Verification items for the finished model (mm, model axes). Face numbers are marked on the shaded views. A direction names the side the tool comes from. Round coordinates to 2 decimals unless told otherwise and drop trailing zeros. Loops run counter-clockwise (first coordinate to the right, second up) from the corner with the lowest first, then second, coordinate; pieces in that order, holes last.
from build123d import *

# Parameters (mm, degrees)
F3_DEPTH = 0.2
F5_COUNT = 4


# Not quite as in the source:
# - a feature of the source that left no trace in its solid (it failed there, or was rolled back) is left out


with BuildPart() as f1:
    # F0 (on Front) → F1 (revolve)
    with BuildSketch(Plane.XZ):
        with BuildLine():
            Line((0, 19.7916666667), (0, 0))
            Line((0, 0), (0.4409722222, 0))
            Line((0.4409722222, 0), (0.4409722222, 19.4444444444))
            Line((0.4409722222, 19.4444444444), (0.3249042511, 19.6180555556))
            ThreePointArc((0.3249042511, 19.6180555556), (0.1841898411, 19.745542126), (0, 19.7916666667))
        make_face()
    revolve(axis=Axis((0, 0, 9.8958333333), (0, 0, 1)))

    # F2 (on Front) → F3 (join, symmetric)
    with BuildSketch(Plane.XZ):
        with BuildLine():
            Line((2.0138888889, 3.2291666667), (0.6493055556, 4.5833333333))
            Line((0.6493055556, 4.5833333333), (-0.6493055556, 4.5833333333))
            Line((-0.6493055556, 4.5833333333), (-2.0138888889, 3.2291666667))
            Line((-2.0138888889, 3.2291666667), (-2.0138888889, 1.2291666667))
            Line((-2.0138888889, 1.2291666667), (-1.875, 1.0902777778))
            Line((-1.875, 1.0902777778), (-1.9722222222, 1.0902777778))
            Line((-1.9722222222, 1.0902777778), (-2.0138888889, 1.0486111111))
            Line((-2.0138888889, 1.0486111111), (-2.0138888889, 0.9930555556))
            ThreePointArc((-2.0138888889, 0.9930555556), (-2.1527777778, 0.7673611111), (-2.0138888889, 0.5416666667))
            Line((-2.0138888889, 0.5416666667), (-2.0138888889, 0.4166666667))
            Line((-2.0138888889, 0.4166666667), (2.0138888889, 0.4166666667))
            Line((2.0138888889, 0.4166666667), (2.0138888889, 0.5416666667))
            ThreePointArc((2.0138888889, 0.5416666667), (2.1527777778, 0.7673611111), (2.0138888889, 0.9930555556))
            Line((2.0138888889, 0.9930555556), (2.0138888889, 1.0486111111))
            Line((2.0138888889, 1.0486111111), (1.9722222222, 1.0902777778))
            Line((1.9722222222, 1.0902777778), (1.875, 1.0902777778))
            Line((1.875, 1.0902777778), (2.0138888889, 1.2291666667))
            Line((2.0138888889, 1.2291666667), (2.0138888889, 3.2291666667))
        make_face()
        with BuildLine():
            Line((0.4409722222, 17.8819444444), (-0.4409722222, 17.8819444444))
            ThreePointArc((-0.4409722222, 17.8819444444), (-0.5180541376, 17.8643461976), (-0.5798611111, 17.8150388148))
            Line((-0.5798611111, 17.8150388148), (-1.1354166667, 17.1180555556))
            Line((-1.1354166667, 17.1180555556), (-1.9632069856, 16.4955808322))
            ThreePointArc((-1.9632069856, 16.4955808322), (-1.9771060186, 16.4509380855), (-1.9391666667, 16.4236111111))
            Line((-1.9391666667, 16.4236111111), (1.9391666667, 16.4236111111))
            ThreePointArc((1.9391666667, 16.4236111111), (1.9771060186, 16.4509380855), (1.9632069856, 16.4955808322))
            Line((1.9632069856, 16.4955808322), (1.1354166667, 17.1180555556))
            Line((1.1354166667, 17.1180555556), (0.5798611111, 17.8150388148))
            ThreePointArc((0.5798611111, 17.8150388148), (0.5180541376, 17.8643461976), (0.4409722222, 17.8819444444))
        make_face()
    extrude(amount=F3_DEPTH, both=True)

    # F5: F1 ×4 about axis
    f5_axis = Axis((0, 0, 0), (0, 0, 1))


with BuildPart() as f1_1:
    add(f1.part)
    for i in range(1, F5_COUNT):
        add(f1.part.rotate(f5_axis, i * 360 / F5_COUNT))


solid = f1_1.part
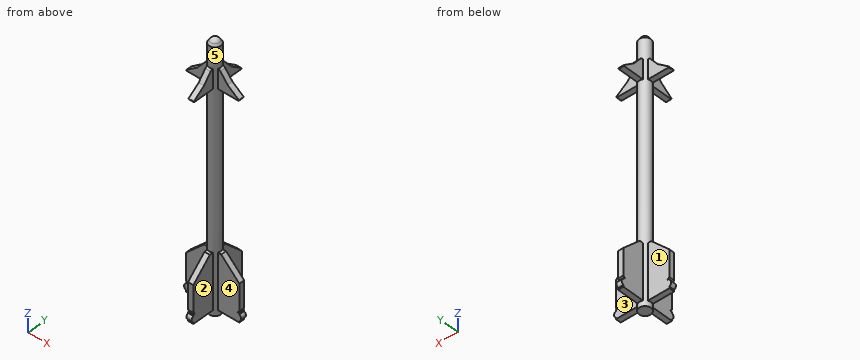
1. Section check B-B (z = 15.5). Enter the section's corners in (x, y).
2. Release check for a two-part mould opening along Z. For the marked faces 4 and 5 record: released by +Z, released by -Z, zero draft, split by the parting line, or undercut.
3. Tool access check on the marked faces 1, 2 and 3. Record the directions out of +Z, -Z, +X, -X, +Y, -Y that give a thin tool (end or side, any length) a straight path to the whole face; none if there is none.
4. Section check A-A (y = 1.65). Enter the section's corners in (x, z), then the cut area to 3 significant figures.
5. Gauge pin test, flat ends, axial feed: P1, Ø1.9, axis at x = -1.5, z = 3.5, coming from the +Y side; P2, Ø1, axis at y = -1, z = 7, coming from the -X side; P3, Ø0.9, axis at y = -1.5, z = 2, coming from the -X side; P4, Ø1, axis at x = -1.5, y = -0.5, coming from the +Z side. Record the tip position at first contact, or that the pin passes through.
6. Scan lines: L1, parallel to X at y = -0.1, z = 3; L2, parallel to Y at x = 0.95, z = 1.5. Record each from-to range of solid material in increasing order.
Taken from the geometry:
1. outline: circle Ø0.88 at (0, 0)
2. face 4: zero draft
2. face 5: undercut
3. face 1: +Z, -Z, -X, +Y
3. face 2: +Z, -Z, +X, -Y
3. face 3: +Z, -Z, +X, +Y
4. outline: (-0.2, 0.42) - (0.2, 0.42) - (0.2, 3.59) - (-0.2, 3.59) - close; (-0.2, 16.42) - (0.2, 16.42) - (0.2, 16.73) - (-0.2, 16.73) - close
4. area: 1.39 mm2
5. P1: stops at y = 0.2
5. P2: passes through
5. P3: stops at x = -0.2
5. P4: stops at z = 17.16
6. L1: x = -2.01 to 2.01
6. L2: y = -0.2 to 0.2
